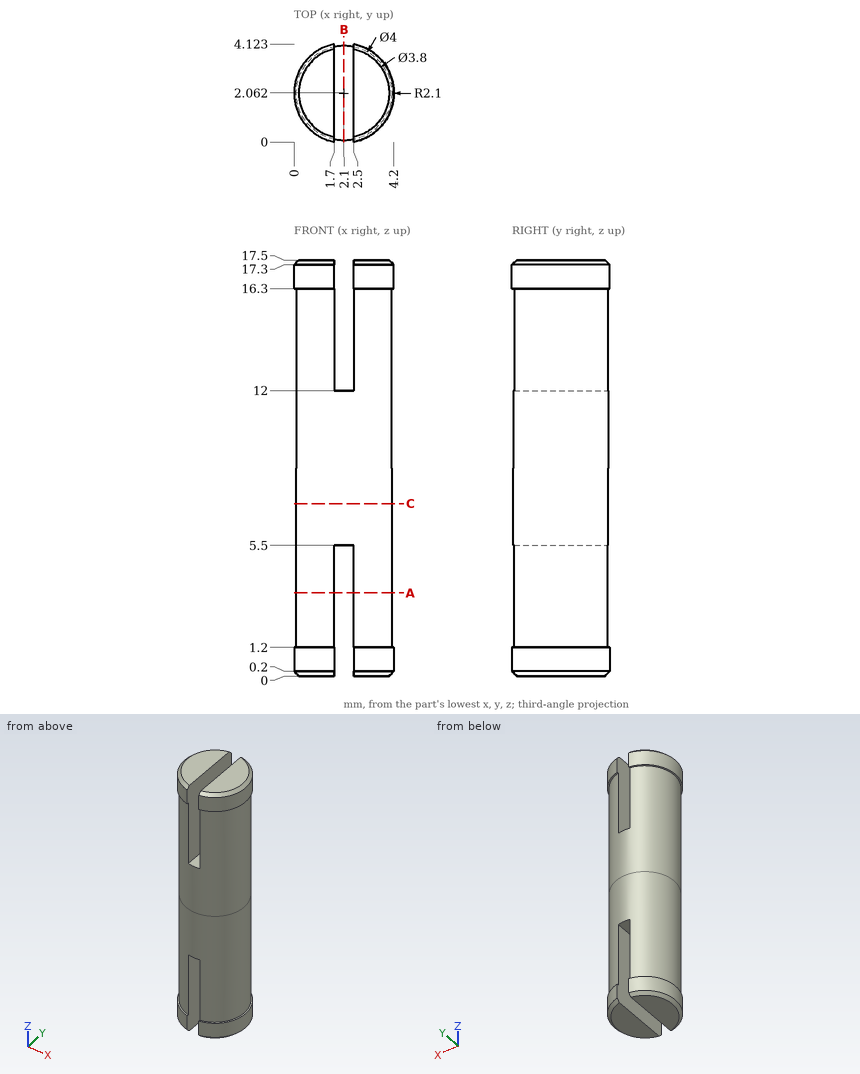
Geometry: see drawing. Coordinates: mm, zero at the bounding-box minimum. Coordinates: 2 decimals unless noted, no trailing zeros. Loops run counter-clockwise (first coordinate to the right, second up) from the corner with the lowest first, then second, coordinate; pieces in that order, holes last. Notation, with made-up numbers: (16, 33) -> (42, 33) arc R23 ccw to (42, 60) -> close; hole circle Ø1 at (55, -7). An arc over 180 degrees is marked (long way). Write item = value, one per line. Start each with the question number.
Item 1: Material intervals for line 1 (X direction, y = 2, z = 7.75); line 2 (Z direction, x = 2.4, y = 2.5); line 3 (X direction, y = 3.15, z = 2.75), sorted ascending.
Item 2: Cut plane B-B, the plane x = 2.1. Return loops of the section in (y, z), plus the area to 3 significant figures.
Item 3: First-contact query: P1, Ø1.2, axis at y = 2, z = 4, coming from the -X side; P2, Ø1.5, axis at y = 2, z = 8, coming from the +X side; P3, Ø1.5, axis at y = 3.5, z = 9.5, coming from the -X side. Flat tips, straight axial feed; report the tip coordinate or a pass-through.
Item 4: Cut plane A-A, the plane z = 3.5. Return loops of the section in (x, y).
Item 5: Cut plane C-C, the plane z = 7.25. Return loops of the section in (x, y), plus the area to 3 significant figures.
Ans:
q1.line_1 = 0.1 to 4.1
q1.line_2 = 5.5 to 12
q1.line_3 = 0.42 to 1.7, 2.5 to 3.78
q2.outline = (0.06, 5.5) -> (4.06, 5.5) -> (4.06, 12) -> (0.06, 12) -> close
q2.area = 26.0 mm²
q3.P1 = 0.1
q3.P2 = 4.1
q3.P3 = 0.22
q4.outline = (1.7, 0.1) -> (1.7, 4.02) arc R2 ccw to start; (2.5, 0.1) arc R2 ccw to (2.5, 4.02) -> close
q5.outline = circle Ø4 at (2.1, 2.06)
q5.area = 12.6 mm²
